Could you check a few things on this model? Use its own coordinates, in mm. A direction names the side the tool comes from. Give positions to 0.01 mm unless a question says otherwise; leave off trailing zeros. Loops run counter-clockwise (first coordinate to the right, second up) from the corner with the lowest first, then second, coordinate; pieces in that order, holes last. Notation, with made-up numbers: M -28,26.5 L 4,26.5 A19 ccw 4,54.5 Z; hole C -21.75,89 d8. An arc over 180 degrees is marked long. Return JSON: item names as keys, results as strings. Group by question number.
1. For pin 1 (1.6 mm diameter, centred on x = 2, z = 24.5, fed in from -Y); pin 2 (2 mm diameter, centred on y = 121.77, z = 82.45, fed in from -X); pin 3 (1.6 mm diameter, centred on x = 2, z = 37.5, fed in from -Y); pin 4 (1.6 mm diameter, centred on x = 2, y = 109.5, fed in from -Z), each with a flat end and sliding along its axis, tell me the tip position at first contact or that it passes through.
2. If we section it at C-C (x = 2.2): State how many separate pieces and enclosed holes the cut face has, plus the area to 3 significant figures.
3. If we section it at A-A (y = 0): Write out the boundary of the cut face in (x, z), plus the area to 3 significant figures.
4. If we section it at B-B (z = 77.68): Write out the boundary of the cut face in (x, y) (3 decimals).
5. Please list where these lines run through material, in increasing order: line 1 (Y direction, x = 0.5, z = 12.5); line 2 (Y direction, x = 0.35, z = 35) (3 decimals); line 3 (Z direction, x = 2.5, y = -13.5).
6. For faces 1 (the flat face through (1.568, 181.902, 29.193)), 2 (the flat face through (1.568, 213.423, 35.343)), 3 (the flat face through (3.18, 105.5, 45.8)), which set-ups out of +Z, -Z, +X, -X, +Y, -Y let a thin tool reach every point of the face, with its end or its side?
7. If we mould it in two halves opening along Z, with no side actions, what happens to faces 4 (the flat face through (1.6, 70.5, 59.6)), 5 (the flat face through (1.568, 95.807, 66.131)), 6 (the flat face through (0, 105.5, 45.8))? For each: +Z half, -Z half, draft (parallel to the pull), parting line (faces both ways), or undercut.
```python
from build123d import *

# Parameters (mm, degrees)
EXTRUDE_BASE_DEPTH         = 3.18
SKETCH4_R                  = 18.5
CUT_MOTOR_HOLES_DEPTH      = 3.18
SKETCH6_R                  = 1.25
SKETCH6_R_2                = 4.765
SUPPORT_HOLES_DEPTH        = 3.18
CUT_LIGHTENING_HOLES_DEPTH = 3.18


with BuildPart() as part:
    # bogie base → extrude-base (new body)
    with BuildSketch(Plane.YZ):
        with BuildLine():
            Line((124.870587973, 92.088866631), (14.608385018, 26.202959511))
            ThreePointArc((14.608385018, 26.202959511), (-25.75271229, -15.388236082), (29.9966211, 0.450247222))
            Line((29.9966211, 0.450247222), (124.870587973, 57.141091426))
            ThreePointArc((124.870587973, 57.141091426), (130, 58.556853997), (135.129412027, 57.141091426))
            Line((135.129412027, 57.141091426), (230.0033789, 0.450247222))
            ThreePointArc((230.0033789, 0.450247222), (285.75271229, -15.388236082), (245.391614982, 26.202959511))
            Line((245.391614982, 26.202959511), (135.129412027, 92.088866631))
            ThreePointArc((135.129412027, 92.088866631), (130, 93.504629201), (124.870587973, 92.088866631))
        make_face()
    extrude(amount=EXTRUDE_BASE_DEPTH)

    # Sketch4 → Cut-motor holes (cut)
    with BuildSketch(Plane.YZ):
        with Locations((260, 0)):
            Circle(SKETCH4_R)
        Circle(SKETCH4_R)
    extrude(amount=CUT_MOTOR_HOLES_DEPTH, mode=Mode.SUBTRACT)

    # Sketch6 → support holes (cut)
    with BuildSketch(Plane.YZ):
        with Locations((64.164835578, 52.110380567)):
            Circle(SKETCH6_R)
        with Locations((84.016579298, 36.433714107)):
            Circle(SKETCH6_R)
        with Locations((130, 77.68)):
            Circle(SKETCH6_R_2)
        with Locations((130, 68.17)):
            Circle(SKETCH6_R)
        with Locations((121.77231361, 82.449200841)):
            Circle(SKETCH6_R)
        with Locations((138.248750332, 82.43704307)):
            Circle(SKETCH6_R)
        with Locations((175.983420702, 36.433714107)):
            Circle(SKETCH6_R)
        with Locations((195.835164422, 52.110380567)):
            Circle(SKETCH6_R)
        with Locations((-23.022924787, -13.757083057)):
            Circle(SKETCH6_R)
        with Locations((283.022924787, -13.757083057)):
            Circle(SKETCH6_R)
    extrude(amount=SUPPORT_HOLES_DEPTH, mode=Mode.SUBTRACT)

    # Sketch7 → Cut-lightening holes (cut)
    with BuildSketch(Plane.YZ):
        with BuildLine():
            Line((54.884000108, 41.646401467), (38.03439682, 28.860792879))
            ThreePointArc((38.03439682, 28.860792879), (37.597600164, 28.332915929), (37.441118366, 27.665863577))
            Line((37.441118366, 27.665863577), (37.441118366, 22.734591544))
            ThreePointArc((37.441118366, 22.734591544), (37.849837551, 21.705462697), (38.853259944, 21.237166789))
            Line((38.853259944, 21.237166789), (49.165938422, 20.63209087))
            ThreePointArc((49.165938422, 20.63209087), (50.727348318, 20.966140733), (51.896208282, 22.053962665))
            Line((51.896208282, 22.053962665), (60.398420976, 35.861757183))
            ThreePointArc((60.398420976, 35.861757183), (60.564389902, 36.239537563), (60.621144468, 36.64824604))
            Line((60.621144468, 36.64824604), (60.621144468, 40.036157787))
            ThreePointArc((60.621144468, 40.036157787), (60.245516663, 41.02902594), (59.306761578, 41.524628912))
            Line((59.306761578, 41.524628912), (55.976338764, 41.939943289))
            ThreePointArc((55.976338764, 41.939943289), (55.401440776, 41.900078528), (54.884000108, 41.646401467))
        make_face()
        with BuildLine():
            Line((200.693238422, 41.524628912), (204.023661236, 41.939943289))
            ThreePointArc((204.023661236, 41.939943289), (204.598559224, 41.900078528), (205.115999892, 41.646401467))
            Line((205.115999892, 41.646401467), (221.96560318, 28.860792879))
            ThreePointArc((221.96560318, 28.860792879), (222.402399836, 28.332915929), (222.558881634, 27.665863577))
            Line((222.558881634, 27.665863577), (222.558881634, 22.734591544))
            ThreePointArc((222.558881634, 22.734591544), (222.150162449, 21.705462697), (221.146740056, 21.237166789))
            Line((221.146740056, 21.237166789), (209.939024731, 20.579576362))
            ThreePointArc((209.939024731, 20.579576362), (209.158319783, 20.746601293), (208.573889801, 21.290512259))
            Line((208.573889801, 21.290512259), (199.601579024, 35.861757183))
            ThreePointArc((199.601579024, 35.861757183), (199.435610098, 36.239537563), (199.378855532, 36.64824604))
            Line((199.378855532, 36.64824604), (199.378855532, 40.036157787))
            ThreePointArc((199.378855532, 40.036157787), (199.754483337, 41.02902594), (200.693238422, 41.524628912))
        make_face()
        with BuildLine():
            Line((112.843083605, 70.967653341), (103.290433505, 70.967653341))
            ThreePointArc((103.290433505, 70.967653341), (102.345892271, 70.815080576), (101.497425215, 70.372881245))
            Line((101.497425215, 70.372881245), (89.954993447, 61.768426002))
            ThreePointArc((89.954993447, 61.768426002), (88.773863738, 58.970129198), (90.641401413, 56.574751268))
            Line((90.641401413, 56.574751268), (99.94028895, 52.884470408))
            ThreePointArc((99.94028895, 52.884470408), (101.439958174, 52.698779238), (102.839897564, 53.267689334))
            Line((102.839897564, 53.267689334), (112.662933935, 60.59039901))
            ThreePointArc((112.662933935, 60.59039901), (113.250900477, 61.170535451), (113.658372475, 61.88902659))
            Line((113.658372475, 61.88902659), (115.631530434, 66.861053016))
            ThreePointArc((115.631530434, 66.861053016), (115.324998286, 69.65291282), (112.843083605, 70.967653341))
        make_face()
        with BuildLine():
            Line((146.341627525, 61.88902659), (144.368469566, 66.861053016))
            ThreePointArc((144.368469566, 66.861053016), (144.675001714, 69.65291282), (147.156916395, 70.967653341))
            Line((147.156916395, 70.967653341), (156.709566495, 70.967653341))
            ThreePointArc((156.709566495, 70.967653341), (157.654107729, 70.815080576), (158.502574785, 70.372881245))
            Line((158.502574785, 70.372881245), (170.045006553, 61.768426002))
            ThreePointArc((170.045006553, 61.768426002), (171.226136262, 58.970129198), (169.358598587, 56.574751268))
            Line((169.358598587, 56.574751268), (160.05971105, 52.884470408))
            ThreePointArc((160.05971105, 52.884470408), (158.560041826, 52.698779238), (157.160102436, 53.267689334))
            Line((157.160102436, 53.267689334), (147.337066065, 60.59039901))
            ThreePointArc((147.337066065, 60.59039901), (146.749099523, 61.170535451), (146.341627525, 61.88902659))
        make_face()
    extrude(amount=CUT_LIGHTENING_HOLES_DEPTH, mode=Mode.SUBTRACT)


solid = part.part
```
Answer:
{
 "1": {"pin 1": "stops at y = -18.39", "pin 2": "passes through", "pin 3": "stops at y = 32.18", "pin 4": "stops at z = 47.48"},
 "2": {"separate pieces": "1", "enclosed holes": "16", "area": "9,530 mm²"},
 "3": {"outline": "M 0,-30 L 3.18,-30 L 3.18,-18.5 L 0,-18.5 Z; M 0,18.5 L 3.18,18.5 L 3.18,30 L 0,30 Z", "area": "73.1 mm²"},
 "4": {"outline": "M 0,100.757 L 3.18,100.757 L 3.18,125.235 L 0,125.235 Z; M 0,134.765 L 3.18,134.765 L 3.18,159.243 L 0,159.243 Z"},
 "5": {"line 1": "y = -27.27 to -13.64, 13.64 to 50.16, 209.84 to 246.36, 273.64 to 287.27", "line 2": "y = 29.331 to 46.125, 59.868 to 87.817, 172.183 to 200.132, 213.875 to 230.669", "line 3": "z = -26.79 to -12.65, 12.65 to 26.79"},
 "6": {"face 1": "-Z, +X, -X", "face 2": "+X, -X", "face 3": "+Z, -Z, +X, +Y, -Y"},
 "7": {"face 4": "+Z half", "face 5": "undercut", "face 6": "draft"}
}
